from build123d import *

# Parameters (mm, degrees)
BOSS_EXTRUDE1_DEPTH                         = 3.175
CSK_FOR_10_FLAT_HEAD_SOCKET_CAP_SCR_2_COUNT = 2
CSK_FOR_10_FLAT_HEAD_SOCKET_CAP_SCR_2_PITCH = 12.7
CSK_FOR_10_FLAT_HEAD_SOCKET_CAP_SCR_3_COUNT = 2
CSK_FOR_10_FLAT_HEAD_SOCKET_CAP_SCR_3_PITCH = 12.7
FILLET2_R                                   = 12.7


with BuildPart() as part:
    # Sketch1 → Boss-Extrude1 (new body)
    with BuildSketch(Plane(origin=(0, 0, 0), x_dir=(1, 0, 0), z_dir=(0, 1, 0))):
        Polygon((0, 0), (0, 114.3), (-50.8, 114.3), (-50.8, 12.7), (-35.664729374, 0), align=None)
    extrude(amount=BOSS_EXTRUDE1_DEPTH)

    # Sketch6 → CSK for #10 Flat Head Socket Cap Screw1 (revolve, cut)
    with BuildSketch(Plane(origin=(-25.4, 3.175, -76.2), x_dir=(0, 0, 1), z_dir=(1, 0, 0))):
        Polygon((0, 0), (0, 3.175), (2.5527, 3.175), (2.5527, 3.068032542), (5.2197, 0), align=None)
    csk_for_10_flat_head_socket_cap_screw1 = revolve(axis=Axis((-25.4, 9.525, -76.2), (0, -1, 0)), mode=Mode.SUBTRACT)

    # CSK for _10 Flat Head Socket Cap Scr 2: CSK for #10 Flat Head Socket Cap Screw1 ×2
    with Locations(*[(0, 0, i * CSK_FOR_10_FLAT_HEAD_SOCKET_CAP_SCR_2_PITCH) for i in range(1, CSK_FOR_10_FLAT_HEAD_SOCKET_CAP_SCR_2_COUNT)]):
        add(csk_for_10_flat_head_socket_cap_screw1, mode=Mode.SUBTRACT)

    # CSK for _10 Flat Head Socket Cap Scr 3: CSK for #10 Flat Head Socket Cap Screw1 ×2
    with Locations(*[(0, 0, -i * CSK_FOR_10_FLAT_HEAD_SOCKET_CAP_SCR_3_PITCH) for i in range(1, CSK_FOR_10_FLAT_HEAD_SOCKET_CAP_SCR_3_COUNT)]):
        add(csk_for_10_flat_head_socket_cap_screw1, mode=Mode.SUBTRACT)

    # Fillet2
    fillet2_edges = [part.edges().sort_by_distance(p)[0] for p in [
        (-35.664729374, 1.5875, 0),
        (-50.8, 1.5875, -12.7),
        (-50.8, 1.5875, -114.3),
        (0, 1.5875, -114.3),
        (0, 1.5875, 0),
    ]]
    fillet(fillet2_edges, radius=FILLET2_R)


solid = part.part
The listing builds one solid part. Answer for the finished solid, in the listing's coordinates (mm). Give positions to 0.01 mm unless a question says otherwise; leave off trailing zeros. Loops run counter-clockwise (first coordinate to the right, second up) from the corner with the lowest first, then second, coordinate; pieces in that order, holes last. Notation, with made-up numbers: (21, 44) - (39, 44) arc R3 ccw to (39, 48) - close; hole circle Ø6 at (57, 35.5). An arc over 180 degrees is marked (long way). Write each question's results on one line, items separated by ' | '.
1. Consider probe 1 along Z at (x, y) = (-25.4, 0.05); probe 2 along X at (y, z) = (0.05, -76.2); probe 3 along Z at (x, y) = (-43, 1.5). Determine where each line is inside the solid, lowest interval first. Write a range as from..to.
Resolved:
probe 1: z = -114.3..-91.45, -86.35..-78.75, -73.65..-66.05, -60.95..0 | probe 2: x = -50.8..-27.95, -22.85..0 | probe 3: z = -113.32..-6.16
2. Find section C-C, the plane y = 1.9. Write down the section's boundary in (x, z), then the cut area to 3 significant figures.
Resolved:
outline: (-50.8, -101.6) arc R12.7 ccw to (-38.1, -114.3) - (-12.7, -114.3) arc R12.7 ccw to (0, -101.6) - (0, -12.7) arc R12.7 ccw to (-12.7, 0) - (-31.04, 0) arc R12.7 ccw to (-39.21, -2.97) - (-46.26, -8.89) arc R12.7 ccw to (-50.8, -18.62) - close; hole circle Ø8.22 at (-25.4, -88.9); hole circle Ø8.22 at (-25.4, -76.2); hole circle Ø8.22 at (-25.4, -63.5) | area: 5,440 mm^2
3. Find section A-A, the plane x = -25.4. Write down the section's boundary in (y, z) (3 decimals).
Resolved:
outline: (0, -114.3) - (3.175, -114.3) - (3.175, -94.12) - (0.107, -91.453) - (0, -91.453) - close; (0, -86.347) - (0.107, -86.347) - (3.175, -83.68) - (3.175, -81.42) - (0.107, -78.753) - (0, -78.753) - close; (0, -73.647) - (0.107, -73.647) - (3.175, -70.98) - (3.175, -68.72) - (0.107, -66.053) - (0, -66.053) - close; (0, -60.947) - (0.107, -60.947) - (3.175, -58.28) - (3.175, 0) - (0, 0) - close
4. For a pull along X with two mould halves and no side action, classify faces 1 (the face through (-25.52, 0.3, -91.62)), 2 (the face through (0, 2, -57)), 3 (the face through (-26.2, 0.3, -60.9)), 4 (the face through (-49.577, 1.61, -13.185)) as +X half, -X half, draft (parallel to the pull), parting line (faces both ways), or undercut.
Resolved:
face 1: undercut | face 2: +X half | face 3: undercut | face 4: -X half
5. Find section D-D, the plane x = -44.5. Write down the section's boundary in (y, z) (1 decimal).
Resolved:
outline: (0, -112.6) - (3.2, -112.6) - (3.2, -7.4) - (0, -7.4) - close
6. Flat-ended cylindrical pins translate along their axes: P1, Ø8, axis at x = -25.4, z = -76.2, coming from the +Y side; P2, Ø1.5, axis at x = -39.5, y = 1, coming from the -Z side; P3, Ø2, axis at x = -5.5, z = -87.5, coming from the -Y side. Find the tip coordinate at first contact, or state that the pin passes through.
Resolved:
P1: stops at y = 1.77 | P2: stops at z = -114.28 | P3: stops at y = 0
7. Find section B-B, the plane z = -76.2. Write down the section's boundary in (x, y) (3 decimals), then the cut area to 3 significant figures.
Resolved:
outline: (-50.8, 0) - (-27.953, 0) - (-27.953, 0.107) - (-30.62, 3.175) - (-50.8, 3.175) - close; (-22.847, 0) - (0, 0) - (0, 3.175) - (-20.18, 3.175) - (-22.847, 0.107) - close | area: 137 mm^2
